Geometry check sheet. Reference: the model listing, model coordinates, mm. A direction names the side the tool comes from. Round coordinates to 2 decimals unless told otherwise and drop trailing zeros. Loops run counter-clockwise (first coordinate to the right, second up) from the corner with the lowest first, then second, coordinate; pieces in that order, holes last. Notation, with made-up numbers: (49.25, -22) - (71.25, -22) arc R19 ccw to (71.25, 7) - close; hole circle Ø8 at (58, 1). An arc over 180 degrees is marked (long way). Answer in a Markdown table with one row per item. Add a question column.
Autodesk Inventor part; units mm, degrees
ref_plane "YZ Plane" through (0, 0, 0) normal (1, 0, 0) x (0, 1, 0)
ref_plane "XZ Plane" through (0, 0, 0) normal (0, 1, 0) x (-1, 0, 0)
ref_plane "XY Plane" through (0, 0, 0) normal (0, 0, 1) x (1, 0, 0)
sketch "Sketch1" plane through (0, 0, 0) normal (0, 1, 0) x (-1, 0, 0)
  line L0 (-23, 55) -> (23, 55)
  line L1 (23, 55) -> (23, -55)
  line L2 (23, -55) -> (-23, -55)
  line L3 (-23, -55) -> (-23, 55)
  line L4 (-23, 55) -> (23, -55) construction
  line L5 (23, 55) -> (-23, -55) construction
  point P0 (0, 0)
  dimension "d0" = 46
  dimension "d1" = 110
extrude "Extrusion1" add sketch "Sketch1" along normal blind 3
sketch "Sketch2" plane through (0, 3, 0) normal (0, 1, 0) x (1, 0, 0)
  line L0 (-23, 55) -> (-23, -55)
  line L1 (23, -55) -> (-23, -55)
  line L2 (-23, -55) -> (-23, 55)
  line L3 (-23, 55) -> (23, 55)
  line L4 (23, 55) -> (23, -55)
  line L5 (23, -55) -> (-23, 55) construction
  line L6 (-23, -55) -> (23, 55) construction
  line L7 (21, -53) -> (-21, -53)
  line L8 (-21, -53) -> (-21, 53)
  line L9 (-21, 53) -> (21, 53)
  line L10 (21, 53) -> (21, -53)
  line L11 (21, -53) -> (-21, 53) construction
  line L12 (-21, -53) -> (21, 53) construction
  point P0 (0, 0)
  dimension "d4" = 42
  dimension "d5" = 106
extrude "Extrusion2" add sketch "Sketch2" along normal blind 30
sketch "Sketch5" plane through (0, 33, 0) normal (0, 1, 0) x (1, 0, 0)
  line L0 (23, 55) -> (-23, 55)
  line L1 (23, -55) -> (23, 55)
  line L2 (-23, 55) -> (-23, -55)
  line L3 (21, 53) -> (21, -53)
  line L4 (21, -42) -> (23, -42)
  line L5 (23, -42) -> (23, -3)
  line L6 (23, -3) -> (21, -3)
  line L7 (21, -3) -> (21, -42)
  line L8 (-23, -55) -> (23, -55)
  point P0 (0, 0)
  point P1 (22, -42)
  point P2 (22, -3)
  dimension "d24" = 13
  dimension "d25" = 58
extrude "Extrusion5" cut sketch "Sketch5" against normal blind 18 contours L1 L4 L3 L6
sketch "Sketch6" plane through (23, 0, -55) normal (0, 0, -1) x (-1, 0, 0)
  line L0 (15, 22) -> (31, 22)
  line L1 (31, 22) -> (31, 12)
  line L2 (31, 12) -> (15, 12)
  line L3 (15, 12) -> (15, 22)
  line L4 (46, 0) -> (46, 33)
  line L5 (0, 0) -> (46, 0)
  point P0 (23, 0)
  dimension "d28" = 16
  dimension "d29" = 15
  dimension "d30" = 10
  dimension "d32" = 12
extrude "Extrusion6" cut sketch "Sketch6" against normal blind 15
sketch "Sketch7" plane through (-23, 0, 55) normal (0, 0, 1) x (1, 0, 0)
  line L0 (5, 25) -> (31, 25)
  line L1 (31, 25) -> (31, 15)
  line L2 (31, 15) -> (5, 15)
  line L3 (5, 15) -> (5, 25)
  line L4 (0, 0) -> (0, 33)
  line L5 (0, 0) -> (46, 0)
  point P0 (23, 0)
  dimension "d35" = 5
  dimension "d36" = 10
  dimension "d37" = 15
  dimension "d38" = 26
extrude "Extrusion7" cut sketch "Sketch7" against normal blind 15
sketch "Sketch9" plane through (0, 33, 0) normal (0, 1, 0) x (1, 0, 0)
  circle A0 centre (0, -60) radius 2
  line L0 (-23, -55) -> (23, -55)
  line L1 (4, -55) -> (-4, -55)
  line L2 (-4, -55) -> (-4, -60)
  line L3 (4, -60) -> (4, -55)
  arc A1 (-4, -60) -> (4, -60) centre (0, -60) ccw
  circle A2 centre (0, 60) radius 2
  line L4 (23, 55) -> (-23, 55)
  line L5 (4, 55) -> (-4, 55)
  line L6 (-4, 55) -> (-4, 60)
  line L7 (4, 60) -> (4, 55)
  arc A3 (4, 60) -> (-4, 60) centre (0, 60) ccw
  point P0 (0, 0)
  point P1 (0, -55)
  point P2 (0, -55)
  point P3 (0, 55)
  point P4 (0, 55)
  point P5 (0, 55)
  dimension "d77" = 4
  dimension "d78" = 5
  dimension "d79" = 8
  dimension "d80" = 4
  dimension "d81" = 4
  dimension "d82" = 4
  dimension "d83" = 5
  dimension "d84" = 8
  dimension "d85" = 4
extrude "Extrusion10" add sketch "Sketch9" against normal blind 6
fillet "Fillet2" radius 2 6 edges at (-4, 30, -55) (4, 30, -55) (-4, 30, 55) (4, 30, 55) (0, 27, -55) (0, 27, 55)
sketch "Sketch11" plane through (0, 3, 0) normal (0, 1, 0) x (1, 0, 0)
  circle A0 centre (-17.5, 47.75) radius 1
  circle A1 centre (17.5, 47.75) radius 1
  circle A2 centre (-17.5, -47.75) radius 1
  circle A3 centre (17.5, -47.75) radius 1
  line L0 (-21, 53) -> (-21, -53)
  line L1 (-21, 53) -> (-15, 53)
  line L2 (-15, 53) -> (-15, 46)
  line L3 (-15, 46) -> (-21, 46)
  line L4 (-21, 46) -> (-21, 53)
  line L5 (21, 53) -> (-21, 53)
  line L6 (21, 53) -> (15, 53)
  line L7 (15, 53) -> (15, 46)
  line L8 (15, 46) -> (21, 46)
  line L9 (21, 46) -> (21, 53)
  line L10 (-21, -53) -> (-15, -53)
  line L11 (-15, -53) -> (-15, -46)
  line L12 (-15, -46) -> (-21, -46)
  line L13 (-21, -46) -> (-21, -53)
  line L14 (21, -53) -> (15, -53)
  line L15 (15, -53) -> (15, -46)
  line L16 (15, -46) -> (21, -46)
  line L17 (21, -46) -> (21, -53)
  point P0 (0, 0)
  dimension "d95" = 2
  dimension "d96" = 2
  dimension "d97" = 2
  dimension "d98" = 2
  dimension "d99" = 95.5
  dimension "d100" = 35
  dimension "d101" = 47.75
  dimension "d102" = 17.5
  dimension "d103" = 6
  dimension "d104" = 7
  dimension "d105" = 6
  dimension "d106" = 7
  dimension "d107" = 6
  dimension "d108" = 7
  dimension "d109" = 6
  dimension "d110" = 7
extrude "Extrusion11" add sketch "Sketch11" along normal blind 11
fillet "Fillet6" radius 2 20 edges at (-23, 16.5, -55) (-23, 16.5, 55) (23, 16.5, 55) (23, 16.5, -55) (21, 23.5, -53) (-21, 23.5, -53) (-21, 23.5, 53) (21, 23.5, 53) (15, 8.5, -46) (-15, 8.5, -46) (15, 8.5, 46) (-15, 8.5, 46) (21, 8.5, -46) (15, 8.5, -53) (-15, 8.5, -53) (-21, 8.5, -46) (-21, 8.5, 46) (-15, 8.5, 53) (21, 8.5, 46) (15, 8.5, 53)
properties part number "StereoPiBracket"
Q1. Cross-section at C-C, the plane y = 23.5. Enter the section's corners in (x, z), plus the area to 3 significant figures.
Q2. Depth check by flat-ended pin: P1, Ø6, axis at x = -3.5, y = 5, coming from the +Z side; P2, Ø1.6, axis at x = 18, z = 48, coming from the +Y side; P3, Ø10, axis at x = -2, z = 29.5, coming from the +Y side. Enter the tip coordinate at first touch or a pass-through.
Q3. Set-up check for faces 1 (the flat face through (1, 27, 62)), 2 (the flat face through (4, 30, 59)), 3 (the flat face through (-15, 8, -50)): record each of +Z, -Z, +X, -X, +Y, -Y from which the full face is reachable in a straight line by a thin tool's end or side.
Q4. Release check for a two-part mould opening along X. For faces 4 (the flat face through (-4, 30, -58)), 5 (the flat face through (23, 16, -1)), 6 (the flat face through (0, 9, -55)), 7 (the flat face through (-21, 18, 1)) record: +X half, -X half, draft (parallel to the pull), parting line (faces both ways), or undercut.
Q5. Cross-section at D-D, the plane z = 37.5. Enter the section's corners in (x, y), plus the area to 3 significant figures.
Q6. Cross-section at A-A, the plane y = 17. Enter the section's corners in (x, z).
Q7. Cross-section at B-B, the plane x = 0. State how many separate pieces and enclosed holes the cut face has, plus the area to 3 significant figures.
Q8. Scan lines: line 1 (X direction, y = 6.75, z = -47.75); line 2 (Z direction, x = -17.5, y = 9); line 3 (Z direction, x = 0, y = 30). Record each from-to range of solid material in increasing order. Write a range as from..to.
Check sheet entries:
| question | item | result |
|---|---|---|
| 1 | outline | (-23, -53) arc R2 ccw to (-21, -55) - (21, -55) arc R2 ccw to (23, -53) - (23, 3) - (21, 3) - (21, -51) arc R2 cw to (19, -53) - (-19, -53) arc R2 cw to (-21, -51) - (-21, 51) arc R2 cw to (-19, 53) - (-18, 53) - (-18, 55) - (-21, 55) arc R2 ccw to (-23, 53) - close; (8, 53) - (19, 53) arc R2 cw to (21, 51) - (21, 42) - (23, 42) - (23, 53) arc R2 ccw to (21, 55) - (8, 55) - close |
| 1 | area | 478 mm² |
| 2 | P1 | z = 55 |
| 2 | P2 | y = 14 |
| 2 | P3 | y = 3 |
| 3 | face 1 | +Z, +X, -X, -Y |
| 3 | face 2 | +Z, +X, +Y, -Y |
| 3 | face 3 | +Y |
| 4 | face 4 | -X half |
| 4 | face 5 | +X half |
| 4 | face 6 | draft |
| 4 | face 7 | undercut |
| 5 | outline | (-23, 0) - (23, 0) - (23, 15) - (21, 15) - (21, 3) - (-21, 3) - (-21, 33) - (-23, 33) - close |
| 5 | area | 222 mm² |
| 6 | outline | (-23, -53) arc R2 ccw to (-21, -55) - (-8, -55) - (-8, -53) - (-19, -53) arc R2 cw to (-21, -51) - (-21, 51) arc R2 cw to (-19, 53) - (-18, 53) - (-18, 55) - (-21, 55) arc R2 ccw to (-23, 53) - close; (8, -55) - (21, -55) arc R2 ccw to (23, -53) - (23, 3) - (21, 3) - (21, -51) arc R2 cw to (19, -53) - (8, -53) - close; (8, 53) - (19, 53) arc R2 cw to (21, 51) - (21, 42) - (23, 42) - (23, 53) arc R2 ccw to (21, 55) - (8, 55) - close |
| 7 | separate pieces | 5 |
| 7 | enclosed holes | 0 |
| 7 | area | 472 mm² |
| 8 | line 1 | -23..-18.5, -16.5..-15.02, 15.02..16.5, 18.5..23 |
| 8 | line 2 | -55..-48.75, -46.75..-46, 46..46.75, 48.75..55 |
| 8 | line 3 | -64..-62, -58..-53, 53..58, 62..64 |
